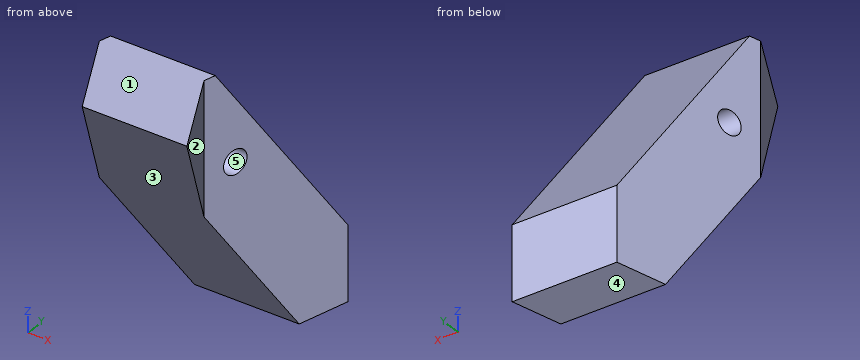
Autodesk Inventor part; units mm, degrees
ref_plane "Work Plane1" through (18.4719, 13.2435, 1) normal (1, 0, 0) x (0, 0, -1)
ref_plane "Work Plane10" through (5.6109, 16.4285, -3.3552) normal (0, -0.829, -0.5592) x (1, 0, 0)
ref_plane "Work Plane11" through (5.6109, 26.377, 3.3552) normal (0, -0.829, -0.5592) x (1, 0, 0)
sketch "Sketch1" plane through (0, 0, 0) normal (0, 0, 1) x (1, 0, 0)
  line L0 (0, 0) -> (5.6109, 21.4027)
  line L1 (5.6109, 21.4027) -> (20.6109, 21.4027)
  line L2 (20.6109, 21.4027) -> (15, 0)
  line L3 (15, 0) -> (21.9438, -13.6515)
  line L4 (21.9438, -13.6515) -> (6.9438, -13.6515)
  line L5 (0, 0) -> (6.9438, -13.6515)
  line L6 (0, 0) -> (0, 15.6682) construction
  dimension "d0" = 138.35
  dimension "d1" = 138.35
  dimension "d2" = 15.316
  dimension "d3" = 22.126
  dimension "d4" = 15
  dimension "d5" = 14.69
extrude "Extrusion1" add sketch "Sketch1" along normal blind 40
ref_plane "Work Plane1" through (18.4719, 13.2435, 1) normal (1, 0, 0) x (0, 0, -1)
sketch "Sketch3" plane through (18.4719, 13.2435, 1) normal (1, 0, 0) x (0, 0, -1)
  circle A0 centre (-25.6667, -8.5907) radius 1.75
  line L0 (1, 8.1593) -> (1, -13.2435)
  line L1 (-39, -13.2435) -> (-39, 8.1593)
  line L2 (1, 8.1593) -> (-39, 8.1593)
  dimension "d11" = 3.5
  dimension "d12" = 26.6667
  dimension "d13" = 13.3333
  dimension "d14" = 15
extrude "Extrusion3" cut sketch "Sketch3" against normal through all
ref_plane "Work Plane9" through (5.6109, 21.4027, 0) normal (0, -0.829, -0.5592) x (1, 0, 0)
ref_plane "Work Plane8" through (21.9438, -13.6515, 40) normal (0, -1, 0) x (1, 0, 0)
ref_plane "Work Plane10" through (5.6109, 16.4285, -3.3552) normal (0, -0.829, -0.5592) x (1, 0, 0)
ref_plane "Work Plane11" through (5.6109, 26.377, 3.3552) normal (0, -0.829, -0.5592) x (1, 0, 0)
split "Split7" plane through (5.6109, 26.377, 3.3552) removes the side toward (0, 0.829, 0.5592)
split "Split8" plane through (5.6109, 16.4285, -3.3552) removes the side toward (0, -0.829, -0.5592)
equation "\"d1\" = d0"
equation "\"d12\" = 2 * d13"
properties part number "Screen Adapter"
Source: CAD feature listing. Evaluate the final solid. Frame: model axes, mm. Face numbers are marked on the shaded views. A direction names the side the tool comes from. Round coordinates to 2 decimals unless told otherwise and drop trailing zeros. Loops run counter-clockwise (first coordinate to the right, second up) from the corner with the lowest first, then second, coordinate; pieces in that order, holes last.
1. Section query D-D on x = 12.25. Output: boundary loops of the cut face in (y, z).
2. Mould query, pull axis Y, two halves, no side actions, for the marked faces 3, 4 and 5. Classes: released by +Y, released by -Y, zero draft, split by the parting line, or undercut.
3. Section query C-C on y = 18. Output: boundary loops of the cut face in (x, z), and give its area (3 significant figures).
4. Ray query, L1, parallel to Y at x = 11.5, z = 17.5; L2, parallel to X at y = -0.5, z = 38; L3, parallel to Y at x = 13.75, z = 10. Return the intervals inside material, ascending.
5. Section query A-A on x = 2.25. Output: boundary loops of the cut face in (y, z).
6. Contact query for flat-ended pins moving along their axis: pin 1 (5 mm diameter, centred on y = 11, z = 15.5, fed in from -X); pin 2 (3 mm diameter, centred on x = 8, z = 27, fed in from -Y); pin 3 (8 mm diameter, centred on y = 14, z = 20.5, fed in from +X); pin 4 (2 mm diameter, centred on y = 4.65, z = 26.67, fed in from +X). Output: stop coordinate, or through.
7. Section query B-B on z = 21.5. Output: boundary loops of the cut face in (x, y).
8. Access query for the marked faces 1 and 2. Directions: +Z, -Z, +X, -X, +Y, -Y. A direction counts if a zero-diameter tool reaches every point of the face in a straight line with its end or side. Return the directions, or none.
Answers below:
1. outline: (-12.81, 40) - (14.17, 0) - (21.4, 0) - (21.4, 10.73) - (1.66, 40) - close; hole circle Ø3.5 at (4.65, 26.67)
2. face 3: released by -Y
2. face 4: zero draft
2. face 5: undercut
3. outline: (4.72, 0) - (19.72, 0) - (19.72, 15.77) - (4.72, 15.77) - close
3. area: 237 mm2
4. L1: y = 2.36 to 16.84
4. L2: x = 0.25 to 15.25
4. L3: y = 7.42 to 21.4
5. outline: (-4.42, 27.56) - (8.58, 8.28) - (8.58, 29.74) - (1.66, 40) - (-4.42, 40) - close; hole circle Ø3.5 at (4.65, 26.67)
6. pin 1: stops at x = 2.23
6. pin 2: stops at y = -5.06
6. pin 3: stops at x = 19.39
6. pin 4: passes through
7. outline: (0, 0) - (0.17, -0.34) - (15.17, -0.34) - (15, 0) - (18.71, 14.14) - (3.71, 14.14) - close
8. face 1: +Z, +X, -X, +Y, -Y
8. face 2: +Z, -Z, +X
